Input: part model. Units: mm. Frame: model coordinates. Face numbers are marked on the shaded views. A direction names the side the tool comes from. Round coordinates to 2 decimals unless told otherwise and drop trailing zeros. Loops run counter-clockwise (first coordinate to the right, second up) from the corner with the lowest first, then second, coordinate; pieces in that order, holes last.
(1) First-contact query: pin 1 Ø7.5 at (x, y) = (18, 13) entering from -Z; pin 2 Ø3.5 at (y, z) = (12.7, -38.1) entering from -X. Flat tips, straight axial feed; report the tip coordinate or a pass-through.
(2) Cut plane A-A, the plane y = 12.7. Output: boundary loops of the cut face in (x, z) (3 decimals), and give its area (3 significant figures).
(3) Cut plane C-C, the plane y = 3. Output: boundary loops of the cut face in (x, z), and give its area (3 significant figures).
(4) Access query for the marked faces 1 and 2. Directions: +Z, -Z, +X, -X, +Y, -Y. A direction counts if a zero-diameter tool reaches every point of the face in a straight line with its end or side. Return the directions, or none.
(5) Line query: line 1 (Y direction, x = 26.95, z = -38.1) (3 decimals); line 2 (X direction, y = 17, z = -118.5); line 3 (Z direction, x = 25, y = 20.75). Output: solid intervals per line, ascending.
(6) Cut plane D-D, the plane x = 18.5. Output: boundary loops of the cut face in (y, z).
(7) Cut plane B-B, the plane z = -49. Output: boundary loops of the cut face in (x, y).
(8) Draft query along X for the marked faces 3, 4, 5 and 6. Return one class per face: released by +X, released by -X, zero draft, split by the parting line, or undercut.
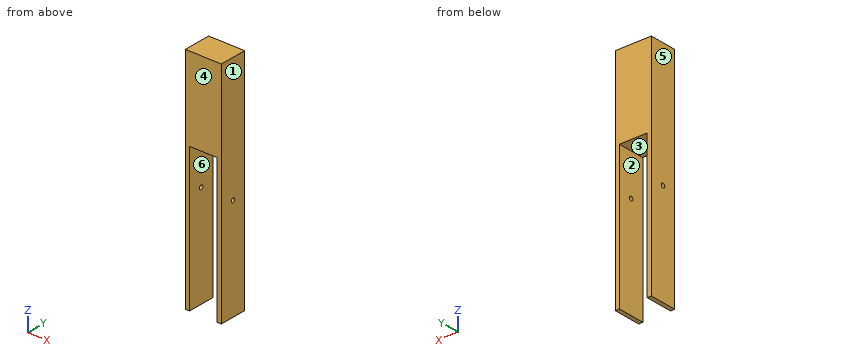
from build123d import *

# Parameters (mm, degrees)
SKETCH2_W           = 25.4
SKETCH2_H           = 25.4
BOSS_EXTRUDE1_DEPTH = 76.2
SKETCH3_W           = 207.924844479
SKETCH3_H           = 25.4
BOSS_EXTRUDE2_DEPTH = 3.81
SKETCH4_W           = 207.924844479
SKETCH4_H           = 25.4
BOSS_EXTRUDE3_DEPTH = 3.81
SKETCH5_R           = 1.905
CUT_EXTRUDE1_DEPTH  = 139.155401824


with BuildPart() as part:
    # Sketch2 → Boss-Extrude1 (new body)
    with BuildSketch(Plane.XY):
        with Locations((12.7, 12.7)):
            Rectangle(SKETCH2_W, SKETCH2_H)
    extrude(amount=BOSS_EXTRUDE1_DEPTH)

    # Sketch3 → Boss-Extrude2 (add)
    with BuildSketch(Plane(origin=(25.4, 0, 0), x_dir=(0, 0, -1), z_dir=(1, 0, 0))):
        with Locations((27.76242224, 12.7)):
            Rectangle(SKETCH3_W, SKETCH3_H)
    extrude(amount=BOSS_EXTRUDE2_DEPTH)

    # Sketch4 → Boss-Extrude3 (add)
    with BuildSketch(Plane.ZY):
        with Locations((-27.76242224, 12.7)):
            Rectangle(SKETCH4_W, SKETCH4_H)
    extrude(amount=BOSS_EXTRUDE3_DEPTH)

    # Sketch5 → Cut-Extrude1 (cut, through all)
    with BuildSketch(Plane.ZY.offset(3.81)):
        with Locations((-38.1, 12.7)):
            Circle(SKETCH5_R)
    extrude(amount=-CUT_EXTRUDE1_DEPTH, mode=Mode.SUBTRACT)


solid = part.part
Reported:
1. pin 1: stops at z = 0
1. pin 2: passes through
2. outline: (-3.81, -131.725) - (0, -131.725) - (0, -40.005) - (-3.81, -40.005) - close; (-3.81, -36.195) - (0, -36.195) - (0, 0) - (25.4, 0) - (25.4, -36.195) - (29.21, -36.195) - (29.21, 76.2) - (-3.81, 76.2) - close; (25.4, -131.725) - (29.21, -131.725) - (29.21, -40.005) - (25.4, -40.005) - close
2. area: 3,490 mm2
3. outline: (-3.81, -131.72) - (0, -131.72) - (0, 0) - (25.4, 0) - (25.4, -131.72) - (29.21, -131.72) - (29.21, 76.2) - (-3.81, 76.2) - close
3. area: 3,520 mm2
4. face 1: +Z, -Z, +X, +Y, -Y
4. face 2: -Z, +Y, -Y
5. line 1: y = 0 to 10.795, 14.605 to 25.4
5. line 2: x = -3.81 to 0, 25.4 to 29.21
5. line 3: z = 0 to 76.2
6. outline: (0, 0) - (25.4, 0) - (25.4, 76.2) - (0, 76.2) - close
7. outline: (-3.81, 0) - (0, 0) - (0, 25.4) - (-3.81, 25.4) - close; (25.4, 0) - (29.21, 0) - (29.21, 25.4) - (25.4, 25.4) - close
8. face 3: undercut
8. face 4: zero draft
8. face 5: released by -X
8. face 6: undercut
